Part model, mm, in its own coordinate system. Face numbers are marked on the shaded views. Give positions to 0.01 mm unless a question says otherwise; leave off trailing zeros. Use one line per item in the form item = value. Start each with the question number.
1. Band-saw the part on A-A, the plane y = -1635. State how many separate pieces and enclosed holes the cut face has, plus the area to 3 significant figures.
2. Pull direction Y, two halves, no side cores. Call the marked faces 1, 2 and 3: +Y half, -Y half, draft (parallel to the pull), parting line (faces both ways), or undercut.
3. Drill centre lines: line 1 (X direction, y = -1981, z = 65); line 2 (X direction, y = -977, z = 122); line 3 (Y direction, x = 421.5, z = 81.5). Where is each one in solid material? Low to high.
4. Pin check, flat tip, straight feed: P1, Ø2.5, axis at y = -2001, z = -29.5, coming from the -X side. Stop position of the tip, or through.
from build123d import *

# Parameters (mm, degrees)
F0_W      = 74
F0_H      = 154
F0_W_2    = 46
F0_H_2    = 46
F1_DEPTH  = 2000
F6_W      = 74
F6_H      = 154
F7_DEPTH  = 582
F8_W      = 74
F8_H      = 154
F9_DEPTH  = 582
F10_W     = 58.25
F10_H     = 30.13
F11_DEPTH = 2160.001
F12_W     = 116.5
F12_H     = 3
F13_DEPTH = 74
F14_W     = 116.5
F14_H     = 3
F15_DEPTH = 76
F16_W     = 116.5
F16_H     = 3
F17_DEPTH = 71
F18_W     = 116.5
F18_H     = 3
F19_DEPTH = 95
F20_W     = 116.5
F20_H     = 3
F20_H_2   = 22.57
F21_DEPTH = 77
F22_DEPTH = 77
F23_DEPTH = 77
F24_W     = 74
F24_H     = 154
F25_DEPTH = 582
F27_DEPTH = 3
F29_DEPTH = 582
F31_DEPTH = 25
F32_DEPTH = 582
F34_DEPTH = 25


# Not quite as in the source:
# - a feature names something its author has since deleted; it is built from what else it names


with BuildPart() as f1:
    # F0 (on Front) → F1 (new body)
    with BuildSketch(Plane.XZ):
        Polygon((-80, 0), (0, 0), (0, 16.85), (0, 31.78), (0, 81.78), (0, 160), (-77, 160), (-80, 160), align=None)
        with Locations((-40, 80)):
            Rectangle(F0_W, F0_H, mode=Mode.SUBTRACT)
        Polygon((0, 81.78), (0, 31.78), (50, 31.78), (50, 81.78), (2, 81.78), align=None)
        with Locations((25, 56.78)):
            Rectangle(F0_W_2, F0_H_2, mode=Mode.SUBTRACT)
    extrude(amount=F1_DEPTH)


with BuildPart() as f2_1:
    # F2: instance of F1
    add(f1.part.mirror(Plane(origin=(50, -1000, 56.78), x_dir=(0, 1, 0), z_dir=(1, 0, 0))))


with BuildPart() as f2_1_1:
    # F3: moved
    add(f2_1.part.moved(Location((63, 0, 0))))


with BuildPart() as f2_1_2:
    # F5: moved
    add(f2_1_1.part.moved(Location((259.1, 0, 0))))


with BuildPart() as f1_1:
    add(f1.part)

    add(f2_1_2.part)  # F7 merges F2_1
    # F6 (on face) → F7 (join)
    with BuildSketch(Plane.YZ.offset(502.1)):
        Polygon((-2000, 0), (-2000, 160), (-2077, 160), (-2080, 160), (-2080, 0), align=None)
        with Locations((-2040, 80)):
            Rectangle(F6_W, F6_H, mode=Mode.SUBTRACT)
    extrude(amount=-F7_DEPTH)

    # F8 (on face) → F9 (join)
    with BuildSketch(Plane.YZ.offset(502.1)):
        Polygon((80, 160), (0, 160), (0, 0), (3, 0), (80, 0), align=None)
        with Locations((40, 80)):
            Rectangle(F8_W, F8_H, mode=Mode.SUBTRACT)
    extrude(amount=-F9_DEPTH)

    # F10 (on face) → F11 (cut, through all)
    with BuildSketch(Plane.XZ.offset(2080)):
        with Locations((182.125, 15.065)):
            Rectangle(F10_W, F10_H)
        with Locations((240.375, 15.065)):
            Rectangle(F10_W, F10_H)
    extrude(amount=-F11_DEPTH, mode=Mode.SUBTRACT)

    # F12 (on face) + F10 (on face) → F13 (join)
    with BuildSketch(Plane(origin=(0, -2077, 0), x_dir=(-1, 0, 0), z_dir=(0, 1, 0))):
        with Locations((-211.25, 31.63)):
            Rectangle(F12_W, F12_H)
    with BuildSketch(Plane.XZ.offset(2080)):
        with Locations((182.125, 15.065)):
            Rectangle(F10_W, F10_H)
    extrude(amount=F13_DEPTH, dir=(0, 1, 0))

    # F14 (on face) → F15 (join)
    with BuildSketch(Plane.XZ.offset(-77)):
        with Locations((211.25, 31.63)):
            Rectangle(F14_W, F14_H)
    extrude(amount=F15_DEPTH)

    # F16 (on face) → F17 (join)
    with BuildSketch(Plane(origin=(0, 0, 30.13), x_dir=(1, 0, 0), z_dir=(0, 0, -1))):
        with Locations((211.25, 2001.5)):
            Rectangle(F16_W, F16_H)
    extrude(amount=F17_DEPTH)

    # F18 (on face) → F19 (join)
    with BuildSketch(Plane(origin=(0, 0, 30.13), x_dir=(1, 0, 0), z_dir=(0, 0, -1))):
        with Locations((211.25, -1.5)):
            Rectangle(F18_W, F18_H)
    extrude(amount=F19_DEPTH)

    # F20 (on face) → F21 (cut)
    with BuildSketch(Plane(origin=(0, 80, 0), x_dir=(-1, 0, 0), z_dir=(0, 1, 0))):
        with Locations((-211.25, 54.2)):
            Rectangle(F20_W, F20_H)
        with Locations((-211.25, 41.415)):
            Rectangle(F20_W, F20_H_2)
    extrude(amount=-F21_DEPTH, mode=Mode.SUBTRACT)

    # F20 (on face) → F22 (join)
    with BuildSketch(Plane(origin=(0, 80, 0), x_dir=(-1, 0, 0), z_dir=(0, 1, 0))):
        with Locations((-211.25, 54.2)):
            Rectangle(F20_W, F20_H)
    extrude(amount=-F22_DEPTH)

    # F10 (on face) → F23 (cut)
    with BuildSketch(Plane.XZ.offset(2080)):
        with Locations((182.125, 15.065)):
            Rectangle(F10_W, F10_H)
    extrude(amount=-F23_DEPTH, mode=Mode.SUBTRACT)

    # F24 (on face) → F25 (join)
    with BuildSketch(Plane(origin=(-79.9, 0, 0), x_dir=(0, -1, 0), z_dir=(-1, 0, 0))):
        Polygon((-80, 3), (-80, 160), (-160, 160), (-160, 0), (-80, 0), align=None)
        with Locations((-120, 80)):
            Rectangle(F24_W, F24_H, mode=Mode.SUBTRACT)
    extrude(amount=-F25_DEPTH)

    # F26 (on face) → F27 (join)
    with BuildSketch(Plane(origin=(0, 160, 0), x_dir=(-1, 0, 0), z_dir=(0, 1, 0))):
        Polygon((-268.7456309795, 160), (-268.7456309795, 0), (-268.7456309795, -64.9877786636), (-152.2456309795, -64.9877786636), (-152.2456309795, 160), align=None)
    extrude(amount=F27_DEPTH)

    # F28 (on face) → F29 (join)
    with BuildSketch(Plane.YZ.offset(502.1)):
        Polygon((282, 160), (160, 160), (160, 157), (279, 157), (279, 3), (160, 3), (160, 0), (282, 0), align=None)
    extrude(amount=-F29_DEPTH)

    # F30 (on face) → F31 (cut)
    with BuildSketch(Plane(origin=(0, 0, 0), x_dir=(1, 0, 0), z_dir=(0, 0, -1))):
        with BuildLine():
            ThreePointArc((250.4956309795, -222.5), (238.779902227, -194.2157287525), (210.4956309795, -182.5))
            Line((210.4956309795, -182.5), (210.4956309795, -222.5))
            Line((210.4956309795, -222.5), (210.4956309795, -262.5))
            ThreePointArc((210.4956309795, -262.5), (238.779902227, -250.7842712475), (250.4956309795, -222.5))
        make_face()
        with BuildLine():
            Line((210.4956309795, -222.5), (210.4956309795, -182.5))
            ThreePointArc((210.4956309795, -182.5), (170.4956309795, -222.5), (210.4956309795, -262.5))
            Line((210.4956309795, -262.5), (210.4956309795, -222.5))
        make_face()
    extrude(amount=-F31_DEPTH, mode=Mode.SUBTRACT)

    # F28 (on face) → F32 (join)
    with BuildSketch(Plane.YZ.offset(502.1)):
        Polygon((-2080, 157), (-2080, 160), (-2202, 160), (-2202, 0), (-2080, 0), (-2080, 3), (-2199, 3), (-2199, 157), align=None)
    extrude(amount=-F32_DEPTH)

    # F33 (on face) → F34 (cut)
    with BuildSketch(Plane(origin=(0, 0, 0), x_dir=(1, 0, 0), z_dir=(0, 0, -1))):
        with BuildLine():
            ThreePointArc((211.25, 2181), (171.25, 2141), (211.25, 2101))
            Line((211.25, 2101), (211.25, 2181))
        make_face()
        with BuildLine():
            Line((211.25, 2181), (211.25, 2101))
            ThreePointArc((211.25, 2101), (239.5342712475, 2112.7157287525), (251.25, 2141))
            ThreePointArc((251.25, 2141), (239.5342712475, 2169.2842712475), (211.25, 2181))
        make_face()
    extrude(amount=-F34_DEPTH, mode=Mode.SUBTRACT)


solid = f1_1.part
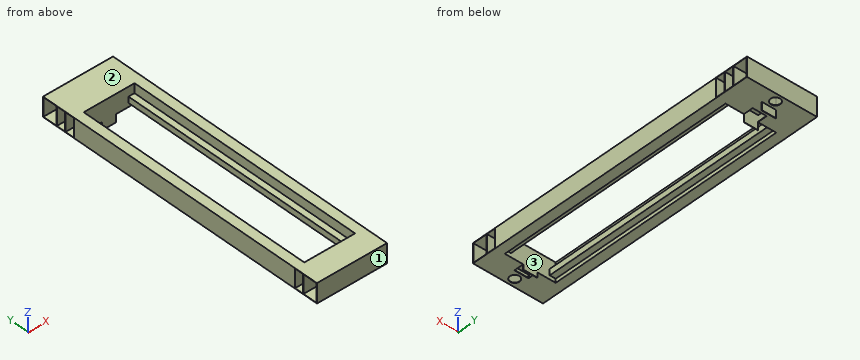
From the geometry:
q1.separate_pieces = 2
q1.enclosed_holes = 4
q1.area = 3,580 mm²
q2.face_1 = -Y half
q2.face_2 = draft
q2.face_3 = undercut
q3.line_1 = -80 to -77, -3 to 2, 48 to 50, 372.1 to 374.1, 420.1 to 425.1, 499.1 to 502.1
q3.line_2 = -80 to -77, -3 to 0, 422.1 to 425.1, 499.1 to 502.1
q3.line_3 = -2202 to -2199, -2080 to -2077, -2003 to 3, 77 to 83, 157 to 160, 279 to 282
q4.P1 = 153
